For this review, use the dimensioned drawing (mm, ordinates from the lowest corner) and the shaded views. Coordinates: 2 decimals unless noted, no trailing zeros. Write each loop counter-clockwise with the first axis right and the second up, starting at its lowest first coordinate (ties: lowest second). Pieces come first, ordered by that corner, then holes. Notation, with made-up numbers: (67.25, -6.75) -> (112.25, -6.75) arc R21 cw to (112.25, 23.25) -> close; hole circle Ø6 at (1, 75.25). An arc over 180 degrees is marked (long way). Put each result on its own line as item: value. Start each with the question number.
Item 1: To check wall thickness, follow L1, parallel to Y at x = 19, z = 1.85. State the ranges of the line that lie inside material, in increasing order.
Item 2: Consider section A-A on x = 167.5. Give the boundary of the cut face in (y, z).
Item 3: Insertion check: P1, Ø3, axis at x = 163.5, z = 2, coming from the +Y side; P2, Ø2, axis at y = 57.5, z = 1.5, coming from the +X side; P3, Ø3, axis at x = 21.5, z = 3, coming from the -Y side. Each pin has a flat end and moves straight along its axis. Give the tip position at first contact, or say it passes through.
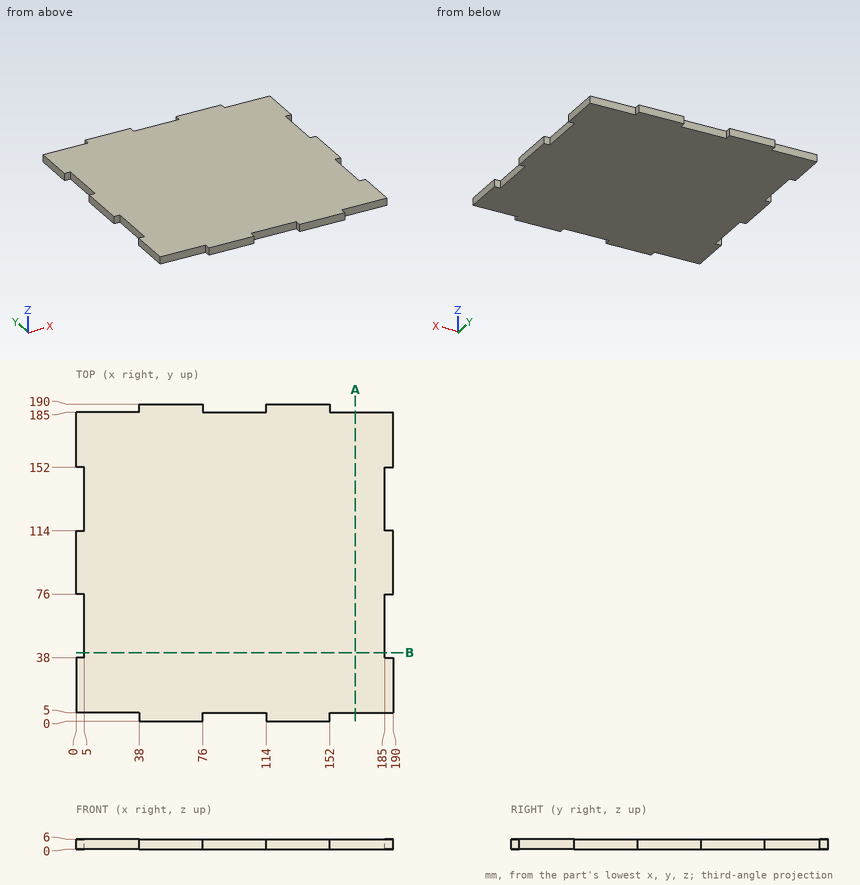
Return value:
1. L1: 5 to 185
2. outline: (5, 0) -> (185, 0) -> (185, 6) -> (5, 6) -> close
3. P1: y = 185
3. P2: x = 185
3. P3: y = 5
